from build123d import *

# Parameters (mm, degrees)
SKETCH_1_W          = 100
SKETCH_1_H          = 45
SKETCH_1_R          = 3
EXTRUDE_1_DEPTH     = 4
SKETCH_2_R          = 1.5
SKETCH_2_R_2        = 2
EXTRUDE_2_DEPTH     = 4
SKETCH_3_W          = 10
SKETCH_3_H          = 15
SKETCH_3_R          = 2
EXTRUDE_3_DEPTH     = 2.4
EXTRUDE_4_DEPTH     = 75
SKETCH_5_R          = 1.5
CUT_EXTRUDE_1_DEPTH = 75
CUT_EXTRUDE_2_DEPTH = 75


with BuildPart() as part:
    # 草图1 → 凸台-拉伸1 (new body)
    with BuildSketch(Plane(origin=(0, 0, 0), x_dir=(1, 0, 0), z_dir=(0, 1, 0))):
        with Locations((50, 22.5)):
            Rectangle(SKETCH_1_W, SKETCH_1_H)
        with Locations((12.5, 35)):
            Circle(SKETCH_1_R, mode=Mode.SUBTRACT)
        with Locations((37.5, 35)):
            Circle(SKETCH_1_R, mode=Mode.SUBTRACT)
        with Locations((37.5, 10)):
            Circle(SKETCH_1_R, mode=Mode.SUBTRACT)
        with Locations((12.5, 10)):
            Circle(SKETCH_1_R, mode=Mode.SUBTRACT)
        with Locations((62.5, 35)):
            Circle(SKETCH_1_R, mode=Mode.SUBTRACT)
        with Locations((62.5, 10)):
            Circle(SKETCH_1_R, mode=Mode.SUBTRACT)
        with Locations((87.5, 10)):
            Circle(SKETCH_1_R, mode=Mode.SUBTRACT)
        with Locations((87.5, 35)):
            Circle(SKETCH_1_R, mode=Mode.SUBTRACT)
    extrude(amount=EXTRUDE_1_DEPTH)

    # 草图2 → 凸台-拉伸2 (add)
    with BuildSketch(Plane.XY):
        Polygon((12.5, 60), (12.5, 0), (87.5, 0), (87.5, 60), (97.5, 60), (97.5, 75), (2.5, 75), (2.5, 60), align=None)
        with Locations((31, 10.5)):
            Circle(SKETCH_2_R, mode=Mode.SUBTRACT)
        with Locations((43, 10.5)):
            Circle(SKETCH_2_R, mode=Mode.SUBTRACT)
        with Locations((57, 10.5)):
            Circle(SKETCH_2_R, mode=Mode.SUBTRACT)
        with Locations((69, 10.5)):
            Circle(SKETCH_2_R, mode=Mode.SUBTRACT)
        with Locations((7.5, 67.5)):
            Circle(SKETCH_2_R_2, mode=Mode.SUBTRACT)
        with Locations((31, 65)):
            Circle(SKETCH_2_R, mode=Mode.SUBTRACT)
        with Locations((69, 65)):
            Circle(SKETCH_2_R, mode=Mode.SUBTRACT)
        with Locations((92.5, 67.5)):
            Circle(SKETCH_2_R_2, mode=Mode.SUBTRACT)
    extrude(amount=-EXTRUDE_2_DEPTH)

    # 草图3 → 凸台-拉伸3 (add)
    with BuildSketch(Plane.XY):
        with Locations((7.5, 67.5)):
            Rectangle(SKETCH_3_W, SKETCH_3_H)
        with Locations((7.5, 67.5)):
            Circle(SKETCH_3_R, mode=Mode.SUBTRACT)
        with Locations((92.5, 67.5)):
            Rectangle(SKETCH_3_W, SKETCH_3_H)
        with Locations((92.5, 67.5)):
            Circle(SKETCH_3_R, mode=Mode.SUBTRACT)
    extrude(amount=EXTRUDE_3_DEPTH)

    # 草图4 → 凸台-拉伸4 (add)
    with BuildSketch(Plane(origin=(87.5, 0, 0), x_dir=(0, 0, -1), z_dir=(1, 0, 0))):
        Polygon((4, 60), (4, 4), (12.5, 4), align=None)
    extrude(amount=-EXTRUDE_4_DEPTH)

    # 草图5 → 切除-拉伸1 (cut)
    with BuildSketch(Plane.XY):
        with Locations((31, 10.5)):
            Circle(SKETCH_5_R)
        with Locations((43, 10.5)):
            Circle(SKETCH_5_R)
        with Locations((57, 10.5)):
            Circle(SKETCH_5_R)
        with Locations((69, 10.5)):
            Circle(SKETCH_5_R)
    extrude(amount=-CUT_EXTRUDE_1_DEPTH, mode=Mode.SUBTRACT)

    # 草图6 → 切除-拉伸2 (cut)
    with BuildSketch(Plane(origin=(0, 4, 0), x_dir=(1, 0, 0), z_dir=(0, 1, 0))):
        Polygon((12.5, 7), (12.5, 4), (21, 4), (21, 12.5), (14.158312395, 12.5), (12.5, 12.5), align=None)
        Polygon((25, 12.5), (25, 4), (75, 4), (75, 12.5), (64.158312395, 12.5), (60.841687605, 12.5), (39.158312395, 12.5), (35.841687605, 12.5), align=None)
        Polygon((79, 12.5), (79, 4), (87.5, 4), (87.5, 7), (87.5, 12.5), (85.841687605, 12.5), align=None)
    extrude(amount=CUT_EXTRUDE_2_DEPTH, mode=Mode.SUBTRACT)


solid = part.part
Could you check a few things on this model? Use its own coordinates, in mm. A direction names the side the tool comes from. Give positions to 0.01 mm unless a question says otherwise; leave off trailing zeros. Order: outer loops, then holes, each group sorted by start corner. A loop starts at its lowest first (then second) coordinate and runs counter-clockwise, first axis right, second up. Notation, with made-up numbers: (-32, 26) - (3, 26) arc R12 cw to (3, 44) - close; hole circle Ø5 at (16, 1). An arc over 180 degrees is marked (long way). One line per item, written item: value. Start each with the question number.
1. For faces 4 (the face through (75, 25, -7)), 5 (the face through (2.5, 67, -1)), 6 (the face through (84.5, 2, -35.1)), 7 (the face through (12.5, 32, -2)), 8 (the face through (93.575, 69.186, -0.845)), which set-ups out of +Z, -Z, +X, -X, +Y, -Y let a thin tool reach every point of the face, with its end or its side?
2. If I drill on probe 1 along X at (y, z) = (65, -2.4); probe 2 along X at (y, z) = (2.5, -10); probe 3 along Y at (x, z) = (69, -3.2), over which ranges is the centre line in solid material (lowest first)?
3. Thinking about a two-plate mould opening in X: for faces 1 (the face through (21, 25, -7)), 2 (the face through (6.3, 69.3, 2.4)), 3 (the face through (25, 19, -6)), which applies, +X half, -X half, draft (parallel to the pull), parting line (faces both ways), or undercut?
4. For P1, Ø1.9, axis at y = 71, z = -0.5, coming from the +X side; P2, Ø8, axis at x = 86.5, z = -8.5, coming from the +Y side; P3, Ø2, axis at y = 21, z = -2.5, coming from the +X side, each with a flat end and sliding along its axis, tell me the tip position at first contact or that it passes through.
5. Imagine slicing it at D-D on y = 38.5. List the corners of the cut face in (x, z) for me.
6. Imagine slicing it at A-A on x = 37.5. List the corners of the cut face in (y, z) for me, plus the area to 3 significant figures.
7. Imagine slicing it at B-B on x = 57. List the corners of the cut face in (y, z) for me, plus the area to 3 significant figures.
8. Imagine slicing it at C-C on x = 23. List the corners of the cut face in (y, z) for me, plus the area to 3 significant figures.
Values:
1. face 4: -Z, +Y
1. face 5: +Z, -Z, -X, +Y
1. face 6: +Y, -Y
1. face 7: +Z, -Z, -X
1. face 8: +Z, -Z
2. probe 1: 2.5 to 29.5, 32.5 to 67.5, 70.5 to 97.5
2. probe 2: 0 to 9.5, 15.5 to 34.5, 40.5 to 59.5, 65.5 to 84.5, 90.5 to 100
2. probe 3: 0 to 9, 12 to 63.5, 66.5 to 75
3. face 1: -X half
3. face 2: draft
3. face 3: undercut
4. P1: x = 97.5
4. P2: y = 4
4. P3: x = 87.5
5. outline: (12.5, -4) - (21, -4) - (21, -7.26) - (25, -7.26) - (25, -4) - (75, -4) - (75, -7.26) - (79, -7.26) - (79, -4) - (87.5, -4) - (87.5, 0) - (12.5, 0) - close
6. outline: (0, -45) - (4, -45) - (4, -38) - (0, -38) - close; (0, -32) - (4, -32) - (4, -13) - (0, -13) - close; (0, -7) - (4, -7) - (4, -4) - (75, -4) - (75, 0) - (0, 0) - close
6. area: 416 mm²
7. outline: (0, -45) - (4, -45) - (4, -4) - (9, -4) - (9, 0) - (0, 0) - close; (12, -4) - (75, -4) - (75, 0) - (12, 0) - close
7. area: 452 mm²
8. outline: (0, -45) - (4, -45) - (4, -12.5) - (60, -4) - (75, -4) - (75, 0) - (0, 0) - close
8. area: 702 mm²
